Here's how the part is built. I have some questions about the finished solid (model axes, mm). A direction names the side the tool comes from. Coordinates: 2 decimals unless noted, no trailing zeros. Order: outer loops, then holes, each group sorted by start corner. A loop starts at its lowest first (then second) coordinate and runs counter-clockwise, first axis right, second up. Notation, with made-up numbers: (15.5, -7.5) - (61.5, -7.5) arc R18 ccw to (61.5, 26.5) - close; hole circle Ø6 at (15, -40). An arc over 180 degrees is marked (long way). Answer as CSV lines item,"result". Start each with the question number.
Item 1: Imagine slicing it at B-B on y = -56.5. Count the separate pieces of the cut face and the enclosed holes in it, and give its area (3 significant figures).
Item 2: Imagine slicing it at D-D on z = -280. List the corners of the cut face in (x, y) for me.
Item 3: I need wall thicknesses on line 1 (Z direction, x = 0, y = -70.5); line 2 (X direction, y = -94, z = -213); line 3 (X direction, y = -142, z = -9.5). Which ranges of each line are inside material? Lowest first, please.
Item 4: Imagine slicing it at C-C on x = 290. List the corners of the cut face in (y, z) for me, and give its area (3 significant figures).
Item 5: I'm going to push flat-ended pins straight in: pin 1 (8 mm diameter, centred on x = 179, y = -99.5, fed in from +Z); pin 2 (10 mm diameter, centred on x = -173, z = 12, fed in from -Y). Where does each tip first touch, or does it pass through?
Item 6: Imagine slicing it at A-A on x = 10.5. List the corners of the cut face in (y, z) for me, and give its area (3 significant figures).
Item 7: On a 3-axis mill with a long thin cutter (end or side, diameter ignored), from which of +Z, -Z, +X, -X, +Y, -Y can I reach the whole of each face in a straight line? I mean faces 1 (the face through (227, -150, -239)), 2 (the face through (-13.77, -49.3, -61.99)). Say none if no direction works.
from build123d import *
from build123d.topology import SkipClean

# Parameters (mm, degrees)
SKETCH1_R                = 350
BOSS_EXTRUDE1_DEPTH      = 5
SKETCH3_R                = 62.5
CUT_EXTRUDE2_DEPTH       = 496
SKETCH2_R                = 40
CUT_EXTRUDE1_DEPTH       = 5
SURFACE_EXTRUDE2_1_DEPTH = 150
THICKEN2_T2              = 1
CIRPATTERN4_COUNT        = 8
CIRPATTERN6_COUNT        = 8
SURFACE_EXTRUDE3_2_DEPTH = 100
THICKEN3_T2              = 1


with BuildPart() as part:
    # Sketch1 → Boss-Extrude1 (new body)
    with BuildSketch(Plane(origin=(0, 0, 0), x_dir=(1, 0, 0), z_dir=(0, 1, 0))):
        with Locations(Location((0, 0, 0), (0, 0, 270))):
            Circle(SKETCH1_R)
    extrude(amount=BOSS_EXTRUDE1_DEPTH)

    # Sketch3 → Cut-Extrude2 (cut, through all)
    with BuildSketch(Plane(origin=(0, 5, 0), x_dir=(1, 0, 0), z_dir=(0, 1, 0))):
        with Locations(Location((0, 0, 0), (0, 0, 270))):
            Circle(SKETCH3_R)
    extrude(amount=-CUT_EXTRUDE2_DEPTH, mode=Mode.SUBTRACT)

    # Sketch2 → Cut-Extrude1 (cut)
    with BuildSketch(Plane(origin=(0, 5, 0), x_dir=(1, 0, 0), z_dir=(0, 1, 0))):
        with Locations(Location((0, 290, 0), (0, 0, 270))):
            Circle(SKETCH2_R)
    cut_extrude1 = extrude(amount=-CUT_EXTRUDE1_DEPTH, mode=Mode.SUBTRACT)

    # Surface-Extrude2: a surface, the sketch's curves swept straight by 150 mm
    with SkipClean():  # the faces are left unmerged after this step: merging them gives an invalid solid
        with BuildLine(Plane.XZ, mode=Mode.PRIVATE) as surface_extrude2_1_path:
            CenterArc((0, -290), 40, 0, 360)
        surface_extrude2_1 = Shell.extrude(surface_extrude2_1_path.wire(), (0 * SURFACE_EXTRUDE2_1_DEPTH, -1 * SURFACE_EXTRUDE2_1_DEPTH, 0 * SURFACE_EXTRUDE2_1_DEPTH))
        add(Solid.thicken(surface_extrude2_1, -THICKEN2_T2))

    # CirPattern4: Cut-Extrude1 ×8 about axis
    with SkipClean():  # the faces are left unmerged after this step: merging them gives an invalid solid
        cirpattern4_axis = Axis((0, 5, 0), (0, 1, 0))
        for i in range(1, CIRPATTERN4_COUNT):
            add(cut_extrude1.rotate(cirpattern4_axis, i * 360 / CIRPATTERN4_COUNT), mode=Mode.SUBTRACT)


with BuildPart() as cirpattern6_1:
    # CirPattern6: pattern copy
    add(part.part.rotate(Axis((0, 0, 0), (0, 1, 0)), 1 * 360 / CIRPATTERN6_COUNT))


with BuildPart() as cirpattern6_2:
    # CirPattern6: pattern copy
    add(part.part.rotate(Axis((0, 0, 0), (0, 1, 0)), 2 * 360 / CIRPATTERN6_COUNT))


with BuildPart() as cirpattern6_3:
    # CirPattern6: pattern copy
    add(part.part.rotate(Axis((0, 0, 0), (0, 1, 0)), 3 * 360 / CIRPATTERN6_COUNT))


with BuildPart() as cirpattern6_4:
    # CirPattern6: pattern copy
    add(part.part.rotate(Axis((0, 0, 0), (0, 1, 0)), 4 * 360 / CIRPATTERN6_COUNT))


with BuildPart() as cirpattern6_5:
    # CirPattern6: pattern copy
    add(part.part.rotate(Axis((0, 0, 0), (0, 1, 0)), 5 * 360 / CIRPATTERN6_COUNT))


with BuildPart() as cirpattern6_6:
    # CirPattern6: pattern copy
    add(part.part.rotate(Axis((0, 0, 0), (0, 1, 0)), 6 * 360 / CIRPATTERN6_COUNT))


with BuildPart() as cirpattern6_7:
    # CirPattern6: pattern copy
    add(part.part.rotate(Axis((0, 0, 0), (0, 1, 0)), 7 * 360 / CIRPATTERN6_COUNT))


with BuildPart() as part_1:
    with SkipClean():  # the faces are left unmerged after this step: merging them gives an invalid solid
        add(part.part)

        add(cirpattern6_1.part)  # Thicken3 merges CirPattern6_1

        add(cirpattern6_2.part)  # Thicken3 merges CirPattern6_2

        add(cirpattern6_3.part)  # Thicken3 merges CirPattern6_3

        add(cirpattern6_4.part)  # Thicken3 merges CirPattern6_4

        add(cirpattern6_5.part)  # Thicken3 merges CirPattern6_5

        add(cirpattern6_6.part)  # Thicken3 merges CirPattern6_6

        add(cirpattern6_7.part)  # Thicken3 merges CirPattern6_7
        # Surface-Extrude3: a surface, the sketch's curves swept straight by 100 mm
        with BuildLine(Plane.XZ, mode=Mode.PRIVATE) as surface_extrude3_2_path:
            CenterArc((0, 0), 62.5, 0, 360)
        surface_extrude3_2 = Shell.extrude(surface_extrude3_2_path.wire(), (0 * SURFACE_EXTRUDE3_2_DEPTH, -1 * SURFACE_EXTRUDE3_2_DEPTH, 0 * SURFACE_EXTRUDE3_2_DEPTH))
        add(Solid.thicken(surface_extrude3_2, -THICKEN3_T2))


solid = part_1.part
Responses:
1,separate pieces,"9"
1,enclosed holes,"9"
1,area,"2,430 mm^2"
2,outline,"(-210, 0) - (-39.76, 0) - (-39.76, -150) - (-38.73, -150) - (-38.73, 5) - (-210, 5) - close; (38.73, -150) - (39.76, -150) - (39.76, 0) - (210, 0) - (210, 5) - (38.73, 5) - close"
3,line 1,"z = -331 to -330, -250 to -249, -63.5 to -62.5, 62.5 to 63.5, 249 to 250, 330 to 331"
3,line 2,"x = -245.28 to -244.27, -165.86 to -164.84, 164.84 to 165.86, 244.27 to 245.28"
3,line 3,"x = -329.88 to -328.86, -251.14 to -250.12, 250.12 to 251.14, 328.86 to 329.88"
4,outline,"(-150, -41) - (0, -41) - (0, -195.96) - (5, -195.96) - (5, -40) - (-150, -40) - close; (-150, 40) - (5, 40) - (5, 195.96) - (0, 195.96) - (0, 41) - (-150, 41) - close"
4,area,"1,860 mm^2"
5,pin 1,"stops at z = 239.62"
5,pin 2,"stops at y = 0"
6,outline,"(-150, -329.63) - (0, -329.63) - (0, -349.84) - (5, -349.84) - (5, -328.6) - (-150, -328.6) - close; (-150, -251.4) - (5, -251.4) - (5, -61.61) - (-100, -61.61) - (-100, -62.63) - (0, -62.63) - (0, -250.37) - (-150, -250.37) - close; (-150, 250.37) - (0, 250.37) - (0, 62.63) - (-100, 62.63) - (-100, 61.61) - (5, 61.61) - (5, 251.4) - (-150, 251.4) - close; (-150, 328.6) - (5, 328.6) - (5, 349.84) - (0, 349.84) - (0, 329.63) - (-150, 329.63) - close"
6,area,"2,930 mm^2"
7,face 1,"+Z, -Z, +X, -X, -Y"
7,face 2,"-Y"
